Study the drawing (mm; zero at the part's minimum x, y, z) and answer. Coordinates: 2 decimals unless noted, no trailing zeros. Order: outer loops, then holes, each group sorted by start corner. A loop starts at its lowest first (then second) coordinate and runs counter-clockwise, first axis right, second up. Notation, with made-up numbers: M 17,6 L 59,6 A36 cw 59,43 Z; hole C 71.5,51 d9. An arc over 180 degrees is marked long. One line per item, written item: value. Start each with the question number.
Q1. The part is cut by section B-B on x = 3. Give the vertices of the cut face in (y, z), then the cut area to 3 significant figures.
Q2. Straight lines are drawn through the part: line 1 along Z through (x, y) = (94, 0.8); line 2 along X through (y, z) = (1.1, 64); line 3 along Z through (x, y) = (16.5, 10). For each, find the intervals that lie inside material, in ascending order. Write a range as [from, to].
Q3. The part is cut by section C-C on z = 23. Give the vertices of the cut face in (x, y), then the cut area to 3 significant figures.
Q4. Determine the mould class of the marked faces 1, 2 and 3 for opening direction Z: pulls with the +Z half, pulls with the -Z half, needs draft (parallel to the pull), parting line crosses it, or undercut.
Q5. The part is cut by section A-A on y = 13.5. Give the vertices of the cut face in (x, z).
Q6. Each of these flat-tipped pins is pushed along its axis until it touches: pin 1 Ø1.5 at (y, z) = (12, 22.5) entering from +X; pin 2 Ø7 at (x, y) = (33.5, 5.5) entering from -Z; pin 3 Ø3 at (x, z) = (56, 64) entering from -Y; pin 4 Ø5 at (x, z) = (56, 23) entering from +Y. Where does it stop, or does it pass through?
Q7. The part is cut by section D-D on x = 56. Give the vertices of the cut face in (y, z), then the cut area to 3 significant figures.
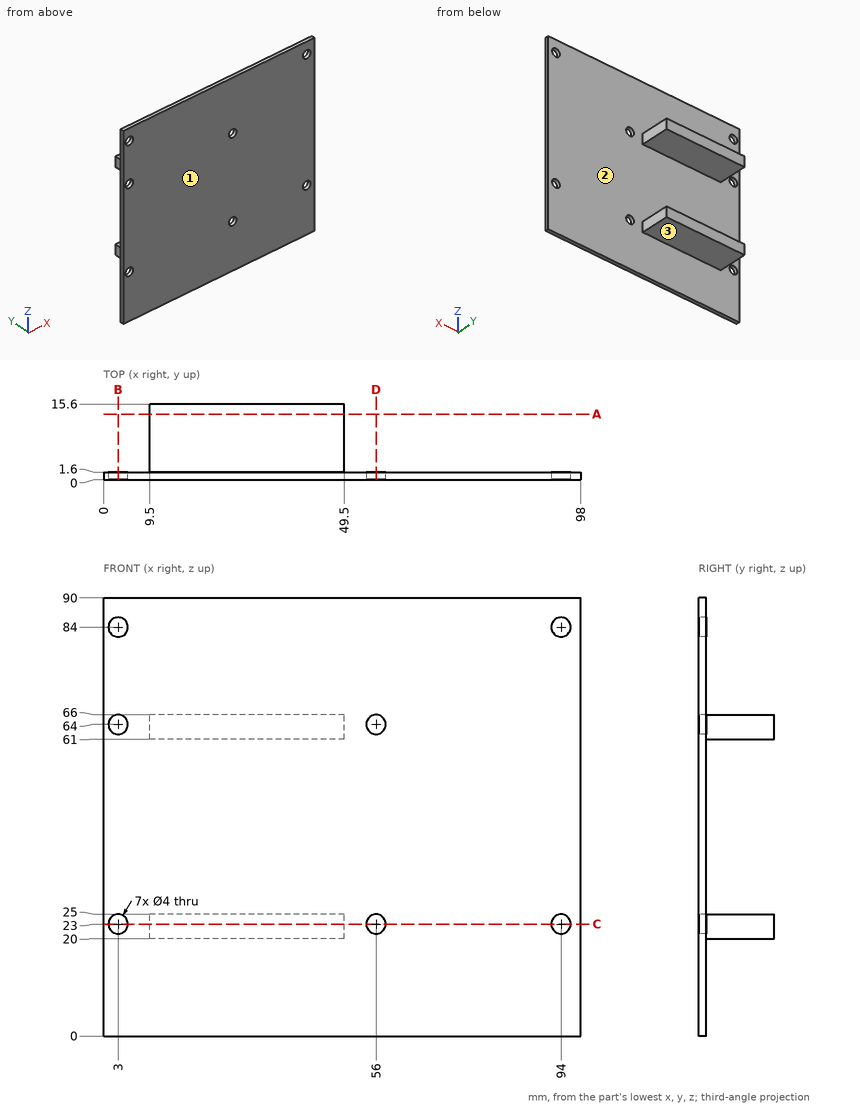
Output:
1. outline: M 0,0 L 1.6,0 L 1.6,21 L 0,21 Z; M 0,25 L 1.6,25 L 1.6,62 L 0,62 Z; M 0,66 L 1.6,66 L 1.6,82 L 0,82 Z; M 0,86 L 1.6,86 L 1.6,90 L 0,90 Z
1. area: 125 mm^2
2. line 1: z = [0, 21], [25, 82], [86, 90]
2. line 2: x = [0, 1], [5, 54], [58, 98]
2. line 3: z = [20, 25], [61, 66]
3. outline: M 0,0 L 1,0 L 1,1.6 L 0,1.6 Z; M 5,0 L 54,0 L 54,1.6 L 49.5,1.6 L 49.5,15.6 L 9.5,15.6 L 9.5,1.6 L 5,1.6 Z; M 58,0 L 92,0 L 92,1.6 L 58,1.6 Z; M 96,0 L 98,0 L 98,1.6 L 96,1.6 Z
3. area: 698 mm^2
4. face 1: needs draft
4. face 2: undercut
4. face 3: pulls with the -Z half
5. outline: M 9.5,20 L 49.5,20 L 49.5,25 L 9.5,25 Z; M 9.5,61 L 49.5,61 L 49.5,66 L 9.5,66 Z
6. pin 1: stops at x = 49.5
6. pin 2: stops at z = 20
6. pin 3: passes through
6. pin 4: stops at y = 1.6
7. outline: M 0,0 L 1.6,0 L 1.6,21 L 0,21 Z; M 0,25 L 1.6,25 L 1.6,62 L 0,62 Z; M 0,66 L 1.6,66 L 1.6,90 L 0,90 Z
7. area: 131 mm^2
